Build history of the part. All positions in model axes, mm. Face numbers are marked on the shaded views. A direction names the side the tool comes from. Give positions to 0.01 mm unless a question says otherwise; leave off trailing zeros. Write each loop counter-clockwise with the first axis right and the second up, starting at its lowest first coordinate (ties: lowest second). Pieces come first, ordered by that corner, then holes. Notation, with made-up numbers: (31, -32.75) -> (50, -32.75) arc R25 ccw to (50, 0.25) -> close; hole circle Ø3 at (-28, 36). An arc over 180 degrees is marked (long way). Write item = value, one per line. Start each with the question number.
Q1. Saw through at B-B, the plane y = 43. List the corners of the cut face in (x, z), then the cut area to 3 significant figures.
Q2. Saw through at A-A, the plane z = 19. List the corners of the cut face in (x, y).
Q3. Wall check: line 1 (Y direction, x = 65.5, z = 37.5); line 2 (Z direction, x = 20, y = 24); line 3 (Y direction, x = 21.5, z = 22.5). Give the ranges that are in metal, low to high.
Q4. Saw through at D-D, the plane z = 28. List the corners of the cut face in (x, y).
Q5. Drop flat-ended pins along their axis: P1, Ø11, axis at y = 42.5, z = 26, coming from the -X side; P2, Ø8, axis at y = 13, z = 16.5, coming from the -X side; P3, Ø3, axis at y = 6, z = 25, coming from the -X side; P4, Ø3, axis at x = 39.5, y = 42, coming from the -Z side. Give the stop position or say it passes through.
Q6. Saw through at C-C, the plane x = 6. List the corners of the cut face in (y, z).
Q7. Mould opens along Y. For the marked faces 1, 2 and 3 say: pulls with the +Y half, pulls with the -Y half, needs draft (parallel to the pull), parting line crosses it, or undercut.
Q8. Tool access for the marked faces 4, 5, 6, 7 and 8: list every direction of +Z, -Z, +X, -X, +Y, -Y with a clear straight run to the whole face (end or side of a thin tool).
from build123d import *

# Parameters (mm, degrees)
SKETCH1_W            = 80
SKETCH1_H            = 50
BOSS_EXTRUDE1_DEPTH  = 10
SKETCH2_W            = 60
SKETCH2_H            = 10
CUT_EXTRUDE1_DEPTH   = 10
CUT_EXTRUDE2_DEPTH   = 10
BOSS_EXTRUDE2_DEPTH  = 10
BOSS_EXTRUDE4_DEPTH  = 40
SKETCH7_W            = 20
SKETCH7_H            = 10
BOSS_EXTRUDE5_DEPTH  = 40
SKETCH8_W            = 40
SKETCH8_H            = 10
BOSS_EXTRUDE6_DEPTH  = 40
BOSS_EXTRUDE7_DEPTH  = 10
BOSS_EXTRUDE8_DEPTH  = 30
BOSS_EXTRUDE9_DEPTH  = 30
BOSS_EXTRUDE11_DEPTH = 20
SKETCH14_W           = 80
SKETCH14_H           = 57.926255319
CUT_EXTRUDE3_DEPTH   = 20
BOSS_EXTRUDE12_DEPTH = 10


with BuildPart() as part:
    # Sketch1 → Boss-Extrude1 (new body)
    with BuildSketch(Plane.XY):
        with Locations((40, 25)):
            Rectangle(SKETCH1_W, SKETCH1_H)
    extrude(amount=BOSS_EXTRUDE1_DEPTH)

    # Sketch2 → Cut-Extrude1 (cut)
    with BuildSketch(Plane.XY.offset(10)):
        with Locations((30, 5)):
            Rectangle(SKETCH2_W, SKETCH2_H)
    extrude(amount=-CUT_EXTRUDE1_DEPTH, mode=Mode.SUBTRACT)

    # Sketch3 → Cut-Extrude2 (cut)
    with BuildSketch(Plane.XY.offset(10)):
        Polygon((40, 10), (0, 30), (0, 10), align=None)
    extrude(amount=-CUT_EXTRUDE2_DEPTH, mode=Mode.SUBTRACT)

    # Sketch4 → Boss-Extrude2 (add)
    with BuildSketch(Plane.XZ):
        Polygon((80, 0), (80, 30), (70, 30), (70, 20), (60, 10), (60, 0), align=None)
    extrude(amount=-BOSS_EXTRUDE2_DEPTH)

    # Sketch6 → Boss-Extrude4 (add)
    with BuildSketch(Plane.XZ.offset(-10)):
        Polygon((40, 10), (80, 10), (80, 40), (60, 40), (40, 30), align=None)
    extrude(amount=-BOSS_EXTRUDE4_DEPTH)

    # Sketch7 → Boss-Extrude5 (add)
    with BuildSketch(Plane.XZ.offset(-10)):
        with Locations((70, 45)):
            Rectangle(SKETCH7_W, SKETCH7_H)
    extrude(amount=-BOSS_EXTRUDE5_DEPTH)

    # Sketch8 → Boss-Extrude6 (add)
    with BuildSketch(Plane.XY.offset(50)):
        with Locations((60, 45)):
            Rectangle(SKETCH8_W, SKETCH8_H)
    extrude(amount=-BOSS_EXTRUDE6_DEPTH)

    # Sketch9 → Boss-Extrude7 (add)
    with BuildSketch(Plane(origin=(0, 40, 0), x_dir=(-1, 0, 0), z_dir=(0, -1, 0))):
        Polygon((-40, -50), (-20, -40), (-20, -23.413516985), (-20, -3.413516985), (-40, -3.413516985), align=None)
    extrude(amount=-BOSS_EXTRUDE7_DEPTH)

    # Sketch10 → Boss-Extrude8 (add)
    with BuildSketch(Plane(origin=(-4, 0, 8), x_dir=(-0.894427191, 0, -0.447213595), z_dir=(0.447213595, 0, -0.894427191))):
        Polygon((-71.55417528, 40), (-71.55417528, 10), (-4.472135955, 30), (-4.472135955, 50), (-49.193495505, 40), align=None)
    extrude(amount=BOSS_EXTRUDE8_DEPTH)

    # Sketch11 → Boss-Extrude9 (add)
    with BuildSketch(Plane(origin=(-4, 0, 8), x_dir=(-0.894427191, 0, -0.447213595), z_dir=(0.447213595, 0, -0.894427191))):
        Polygon((-49.193495505, 10), (-49.193495505, 16.666666667), (-4.472135955, 30), align=None)
    extrude(amount=BOSS_EXTRUDE9_DEPTH)

    # Sketch13 → Boss-Extrude11 (add)
    with BuildSketch(Plane(origin=(12, 24, 0), x_dir=(-0.894427191, 0.447213595, 0), z_dir=(-0.447213595, -0.894427191, 0))):
        Polygon((-31.304951685, -10), (-31.304951685, -30), (13.416407865, -10), align=None)
    extrude(amount=-BOSS_EXTRUDE11_DEPTH)

    # Sketch14 → Cut-Extrude3 (cut)
    with BuildSketch(Plane(origin=(0, 0, 0), x_dir=(-1, 0, 0), z_dir=(0, 0, -1))):
        with Locations((-40, 21.036872341)):
            Rectangle(SKETCH14_W, SKETCH14_H)
    extrude(amount=CUT_EXTRUDE3_DEPTH, mode=Mode.SUBTRACT)

    # Sketch15 → Boss-Extrude12 (add)
    with BuildSketch(Plane(origin=(-4, 0, 8), x_dir=(-0.894427191, 0, -0.447213595), z_dir=(0.447213595, 0, -0.894427191))):
        Polygon((-4.472135955, 50), (-26.83281573, 40), (-26.83281573, 50), align=None)
    extrude(amount=BOSS_EXTRUDE12_DEPTH)


solid = part.part
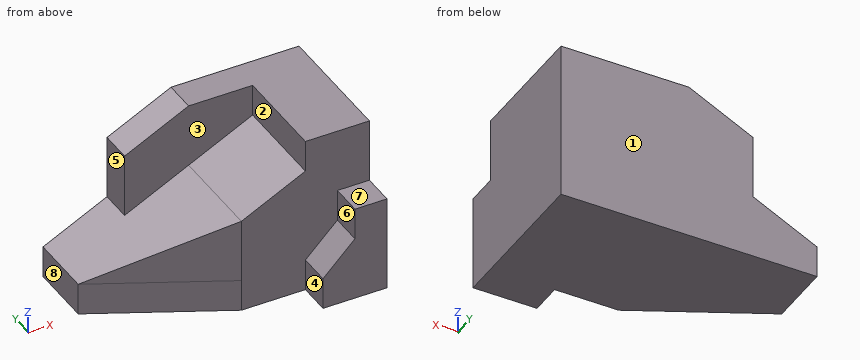
Report:
q1.outline = (0, 0) -> (80, 0) -> (80, 50) -> (40, 50) -> (20, 40) -> (20, 20) -> (0, 10) -> close
q1.area = 3,200 mm2
q2.outline = (18, 21) -> (40, 10) -> (69, 10) -> (69, 0) -> (80, 0) -> (80, 50) -> (18, 50) -> close
q3.line_1 = 10 to 50
q3.line_2 = 0 to 20
q3.line_3 = 40 to 50
q4.outline = (20, 40) -> (36, 40) -> (36, 12) -> (40, 10) -> (70, 10) -> (70, 0) -> (80, 0) -> (80, 50) -> (20, 50) -> close
q5.P1 = 20
q5.P2 = 26
q5.P3 = 70
q5.P4 = 0
q6.outline = (27, 0) -> (50, 0) -> (50, 13) -> (27, 13) -> close
q7.face_1 = pulls with the +Y half
q7.face_2 = needs draft
q7.face_3 = pulls with the -Y half
q8.face_4 = +Z, -Z, -X, -Y
q8.face_5 = +Z, -X, +Y, -Y
q8.face_6 = +Z, -X, -Y
q8.face_7 = +Z, +X, -X, -Y
q8.face_8 = +Z, -Z, -X, +Y, -Y
